Part model, mm, in its own coordinate system. A direction names the side the tool comes from. Coordinates: 2 decimals unless noted, no trailing zeros. Write each loop counter-clockwise with the first axis right and the second up, starting at its lowest first coordinate (ties: lowest second). Pieces come first, ordered by that corner, then holes. Notation, with made-up numbers: M 80.25,-21.5 L 122.25,-21.5 A18 ccw 122.25,-9.5 Z; hole C -32.75,72 d9. An arc over 180 degrees is marked long. Use a Markdown table: item, result. Add a question column.
Q1. Mould opens along X. For faces 5 (the flat face through (-136, 0, 90)), 6 (the flat face through (97.409, -13.944, 14.79)), 7 (the flat face through (75, 0, 60)) say: released by +X, released by -X, zero draft, split by the parting line, or undercut.
Q2. Tool access for faces 1 (the flat face through (97.409, -13.944, 104.79)), 2 (the flat face through (-24, 10, 101)), 3 (the flat face through (-9, 0, 90)), 4 (the flat face through (115, 0, 30)): list every direction of +Z, -Z, +X, -X, +Y, -Y with a clear straight run to the whole face (end or side of a thin tool).
Q3. Slice it at D-D on z = 96. Write the cut outline in (x, y).
Q4. Pin check, flat tips, straight feed: pin 1 Ø25 at (x, y) = (-90, -25.5) entering from -Z; pin 2 Ø16 at (y, z) = (0.5, 60.5) entering from +X; pin 3 Ø1 at (y, z) = (10, 25.5) entering from +X. Stop position of each tip, or through.
Q5. Slice it at C-C on x = -112.5. Write the cut outline in (y, z), then the cut area to 3 significant figures.
Q6. Wall check: L1, parallel to X at y = 0, z = 34; L2, parallel to X at y = 0, z = 23; L3, parallel to Z at x = 37, y = 1. Give the ranges that are in metal, low to high. Write a range as from..to.
Q7. Slice it at B-B on z = 50.5. Write the cut outline in (x, y).
Q8. Slice it at A-A on y = 0. Count the separate pieces of the cut face and the enclosed holes in it, then the cut area to 3 significant figures.
from build123d import *

# Parameters (mm, degrees)
SKETCH1_R           = 10
SKETCH1_R_2         = 15
BOSS_EXTRUDE1_DEPTH = 120
CUT_EXTRUDE1_DEPTH  = 45
SKETCH3_R           = 11
SKETCH3_R_2         = 7.2
BOSS_EXTRUDE2_DEPTH = 120
CUT_EXTRUDE2_DEPTH  = 180
SKETCH5_W           = 31.21991305
SKETCH5_H           = 33.6
BOSS_EXTRUDE3_DEPTH = 20
SKETCH6_W           = 31.21991305
SKETCH6_H           = 20
BOSS_EXTRUDE4_DEPTH = 13.2
SKETCH8_W           = 31.21991305
SKETCH8_H           = 20
BOSS_EXTRUDE5_DEPTH = 13.2
CUT_EXTRUDE3_DEPTH  = 40


with BuildPart() as part:
    # Sketch1 → Boss-Extrude1 (new body)
    with BuildSketch(Plane.XY):
        with BuildLine():
            Line((75, 10), (-124.86381146, 10))
            Line((-124.86381146, 10), (-142.062836025, 19.631407747))
            ThreePointArc((-142.062836025, 19.631407747), (-175.556371847, 0), (-142.062836025, -19.631407747))
            Line((-142.062836025, -19.631407747), (-124.86381146, -10))
            Line((-124.86381146, -10), (75, -10))
            Line((75, -10), (120.453543604, -18.000740708))
            ThreePointArc((120.453543604, -18.000740708), (156.452555937, 0), (120.453543604, 18.000740708))
            Line((120.453543604, 18.000740708), (75, 10))
        make_face()
        with Locations((133.952555937, 0)):
            Circle(SKETCH1_R, mode=Mode.SUBTRACT)
        with Locations((-153.056371847, 0)):
            Circle(SKETCH1_R_2, mode=Mode.SUBTRACT)
    extrude(amount=BOSS_EXTRUDE1_DEPTH)

    # Sketch2 → Cut-Extrude1 (cut, symmetric)
    with BuildSketch(Plane(origin=(0, 10, 0), x_dir=(1, 0, 0), z_dir=(0, 1, 0))):
        Polygon((-124.86381146, -90), (-124.86381146, -60), (-124.86381146, -30), (-189.632147982, -30), (-189.632147982, -90), align=None)
        Polygon((-124.86381146, -30), (-124.86381146, -60), (-124.86381146, -90), (62.44239577, -90), (62.44239577, -30), align=None)
    extrude(amount=CUT_EXTRUDE1_DEPTH, both=True, mode=Mode.SUBTRACT)

    # Sketch3 → Boss-Extrude2 (add)
    with BuildSketch(Plane.XY.offset(120)):
        with BuildLine():
            Line((-109.253854935, -10), (-104.64389841, -47.8166351))
            ThreePointArc((-104.64389841, -47.8166351), (-93.64389841, -36.8166351), (-82.64389841, -47.8166351))
            Line((-82.64389841, -47.8166351), (-78.033941885, -10))
            Line((-78.033941885, -10), (-109.253854935, -10))
        make_face()
        with Locations((-93.64389841, -47.8166351)):
            Circle(SKETCH3_R)
        with Locations((-93.64389841, -47.8166351)):
            Circle(SKETCH3_R_2, mode=Mode.SUBTRACT)
    extrude(amount=-BOSS_EXTRUDE2_DEPTH)

    # Sketch4 → Cut-Extrude2 (cut)
    with BuildSketch(Plane.ZY.offset(-62.44239577)):
        Polygon((43.2, -58.8166351), (43.2, -10), (30, -10), (-9.185341586, -10), (-9.185341586, -58.8166351), align=None)
        Polygon((90, -10), (76.8, -10), (76.8, -58.8166351), (133.966164795, -58.8166351), (133.966164795, -10), align=None)
    extrude(amount=CUT_EXTRUDE2_DEPTH, mode=Mode.SUBTRACT)

    # Sketch5 → Boss-Extrude3 (add)
    with BuildSketch(Plane(origin=(0, -10, 0), x_dir=(1, 0, 0), z_dir=(0, 1, 0))):
        with Locations((-93.64389841, -60)):
            Rectangle(SKETCH5_W, SKETCH5_H)
    extrude(amount=BOSS_EXTRUDE3_DEPTH)

    # Sketch6 → Boss-Extrude4 (add)
    with BuildSketch(Plane(origin=(0, 0, 43.2), x_dir=(-1, 0, 0), z_dir=(0, 0, -1))):
        with Locations((93.64389841, 0)):
            Rectangle(SKETCH6_W, SKETCH6_H)
    extrude(amount=BOSS_EXTRUDE4_DEPTH)

    # Sketch8 → Boss-Extrude5 (add)
    with BuildSketch(Plane(origin=(0, 0, 90), x_dir=(-1, 0, 0), z_dir=(0, 0, -1))):
        with Locations((93.64389841, 0)):
            Rectangle(SKETCH8_W, SKETCH8_H)
    extrude(amount=BOSS_EXTRUDE5_DEPTH)

    # Sketch9 → Cut-Extrude3 (cut, symmetric)
    with BuildSketch(Plane(origin=(0, 10, 0), x_dir=(1, 0, 0), z_dir=(0, 1, 0))):
        Polygon((156.452555937, -30), (156.452555937, -60), (156.452555937, -90), (75, -90), (75, -30), align=None)
    extrude(amount=CUT_EXTRUDE3_DEPTH, both=True, mode=Mode.SUBTRACT)


solid = part.part
Recorded:
| question | item | result |
|---|---|---|
| 1 | face 5 | zero draft |
| 1 | face 6 | undercut |
| 1 | face 7 | released by +X |
| 2 | face 1 | +Z, -Z, -Y |
| 2 | face 2 | +Z, -Z, +Y |
| 2 | face 3 | +Y, -Y |
| 2 | face 4 | +X, +Y, -Y |
| 3 | outline | M -142.06,-19.63 L -124.86,-10 L 75,-10 L 120.45,-18 A22.5 ccw long 120.45,18 L 75,10 L -124.86,10 L -142.06,19.63 A22.5 ccw long Z; hole C -153.06,0 d30; hole C 133.95,0 d20 |
| 4 | pin 1 | z = 43.2 |
| 4 | pin 2 | x = 75 |
| 4 | pin 3 | x = 154.35 |
| 5 | outline | M -10,0 L 10,0 L 10,30 L -10,30 Z; M -10,90 L 10,90 L 10,120 L -10,120 Z |
| 5 | area | 1,200 mm² |
| 6 | L1 | -109.25..-78.03, 62.44..75 |
| 6 | L2 | -175.56..-168.06, -138.06..123.95, 143.95..156.45 |
| 6 | L3 | 0..30, 90..120 |
| 7 | outline | M -109.25,-10 L -104.64,-47.82 A11 ccw -82.64,-47.82 L -78.03,-10 L -78.03,10 L -109.25,10 Z; M 62.44,-10 L 75,-10 L 75,10 L 62.44,10 Z; hole C -93.64,-47.82 d14.4 |
| 8 | separate pieces | 5 |
| 8 | enclosed holes | 1 |
| 8 | area | 19,500 mm² |
